The listing builds one solid part. Answer for the finished solid, in the listing's coordinates (mm). A direction names the side the tool comes from. Round coordinates to 2 decimals unless told otherwise and drop trailing zeros. Order: outer loops, then holes, each group sorted by start corner. A loop starts at its lowest first (then second) coordinate and runs counter-clockwise, first axis right, second up. Notation, with made-up numbers: (-1.75, 53) -> (55.25, 53) arc R13 cw to (55.25, 65) -> close; hole circle Ø11 at (69.25, 81.5). An arc over 180 degrees is marked (long way). Answer in a Markdown table with one row per item. Add a question column.
```python
from build123d import *

# Parameters (mm, degrees)
BOSS_EXTRUDE1_DEPTH = 6
FILLET1_R           = 10


with BuildPart() as part:
    # Sketch1 → Boss-Extrude1 (new body)
    with BuildSketch(Plane(origin=(0, 0, 0), x_dir=(1, 0, 0), z_dir=(0, 1, 0))):
        with BuildLine():
            Line((-72.831998462, 89.802561211), (-13.029437252, 30))
            Line((-13.029437252, 30), (13.029437252, 30))
            Line((13.029437252, 30), (72.831998462, 89.802561211))
            ThreePointArc((72.831998462, 89.802561211), (89.802561211, 89.802561211), (89.802561211, 72.831998462))
            Line((89.802561211, 72.831998462), (30, 13.029437252))
            Line((30, 13.029437252), (30, -13.029437252))
            Line((30, -13.029437252), (89.802561211, -72.831998462))
            ThreePointArc((89.802561211, -72.831998462), (89.802561211, -89.802561211), (72.831998462, -89.802561211))
            Line((72.831998462, -89.802561211), (13.029437252, -30))
            Line((13.029437252, -30), (-13.029437252, -30))
            Line((-13.029437252, -30), (-72.831998462, -89.802561211))
            ThreePointArc((-72.831998462, -89.802561211), (-89.802561211, -89.802561211), (-89.802561211, -72.831998462))
            Line((-89.802561211, -72.831998462), (-30, -13.029437252))
            Line((-30, -13.029437252), (-30, 13.029437252))
            Line((-30, 13.029437252), (-89.802561211, 72.831998462))
            ThreePointArc((-89.802561211, 72.831998462), (-89.802561211, 89.802561211), (-72.831998462, 89.802561211))
        make_face()
    extrude(amount=BOSS_EXTRUDE1_DEPTH)

    # Fillet1
    fillet1_edges = [part.edges().sort_by_distance(p)[0] for p in [
        (-13.029437252, 3, -30),
        (13.029437252, 3, -30),
        (30, 3, -13.029437252),
        (30, 3, 13.029437252),
        (13.029437252, 3, 30),
        (-13.029437252, 3, 30),
        (-30, 3, 13.029437252),
        (-30, 3, -13.029437252),
    ]]
    fillet(fillet1_edges, radius=FILLET1_R)


solid = part.part
```
1. The part is cut by section B-B (z = -67). Give the vertices of the cut face in (x, y), then the cut area to 3 significant figures.
2. Each of these flat-tipped pins is pushed along its axis until it touches: pin 1 (2 mm diameter, centred on y = 4.5, z = 50, fed in from -X); pin 2 (1.8 mm diameter, centred on y = 1.5, z = 3, fed in from +X); pin 3 (2 mm diameter, centred on y = 3, z = -19, fed in from +X). Where does it stop, or does it pass through?
3. The part is cut by section A-A (x = 79.5). Give the vertices of the cut face in (y, z).
4. The part is cut by section C-C (y = 3.3). Give the vertices of the cut face in (x, z), then the cut area to 3 significant figures.
5. The part is cut by section D-D (x = 21.5). Give the vertices of the cut face in (y, z), then the cut area to 3 significant figures.
6. The mould has two halves that part along X. Classify faces 1 (the cylindrical face through (12.76, 3.04, 30.78)), 2 (the flat face through (0, 6, 6)), 3 (the flat face through (61.76, 2.96, -44.79)): released by +X, released by -X, zero draft, split by the parting line, or undercut.
7. For faces 4 (the flat face through (44, 2.96, -60.97)), 5 (the cylindrical face through (30.78, 3.04, -12.76)), 6 (the flat face through (0, 3, 30)), 7 (the cylindrical face through (-89.6, 3, 90)), 8 (the flat face through (-61.76, 2.96, 44.79)), determine the directions among +Z, -Z, +X, -X, +Y, -Y from which every point of the face is accessible in a straight line to the end or side of a thin tool.
8. Straight lines are drawn through the part: line 1 along X through (y, z) = (5.1, -7); line 2 along X through (y, z) = (2.9, -76). For each, find the intervals that lie inside material, in ascending order.
Report:
| question | item | result |
|---|---|---|
| 1 | outline | (-83.97, 0) -> (-50.03, 0) -> (-50.03, 6) -> (-83.97, 6) -> close; (50.03, 0) -> (83.97, 0) -> (83.97, 6) -> (50.03, 6) -> close |
| 1 | area | 407 mm^2 |
| 2 | pin 1 | stops at x = -67.97 |
| 2 | pin 2 | stops at x = 30 |
| 2 | pin 3 | stops at x = 36.97 |
| 3 | outline | (0, -93.18) -> (6, -93.18) -> (6, -62.53) -> (0, -62.53) -> close; (0, 62.53) -> (6, 62.53) -> (6, 93.18) -> (0, 93.18) -> close |
| 4 | outline | (-89.8, -72.83) arc R12 ccw to (-72.83, -89.8) -> (-15.96, -32.93) arc R10 cw to (-8.89, -30) -> (8.89, -30) arc R10 cw to (15.96, -32.93) -> (72.83, -89.8) arc R12 ccw to (89.8, -72.83) -> (32.93, -15.96) arc R10 cw to (30, -8.89) -> (30, 8.89) arc R10 cw to (32.93, 15.96) -> (89.8, 72.83) arc R12 ccw to (72.83, 89.8) -> (15.96, 32.93) arc R10 cw to (8.89, 30) -> (-8.89, 30) arc R10 cw to (-15.96, 32.93) -> (-72.83, 89.8) arc R12 ccw to (-89.8, 72.83) -> (-32.93, 15.96) arc R10 cw to (-30, 8.89) -> (-30, -8.89) arc R10 cw to (-32.93, -15.96) -> close |
| 4 | area | 12,100 mm^2 |
| 5 | outline | (0, -38.47) -> (6, -38.47) -> (6, 38.47) -> (0, 38.47) -> close |
| 5 | area | 462 mm^2 |
| 6 | face 1 | undercut |
| 6 | face 2 | zero draft |
| 6 | face 3 | released by +X |
| 7 | face 4 | -Z, +Y, -Y |
| 7 | face 5 | +X, +Y, -Y |
| 7 | face 6 | +Z, +Y, -Y |
| 7 | face 7 | +Y, -Y |
| 7 | face 8 | -X, +Y, -Y |
| 8 | line 1 | x = -30 to 30 |
| 8 | line 2 | x = -92.07 to -59.03, 59.03 to 92.07 |
